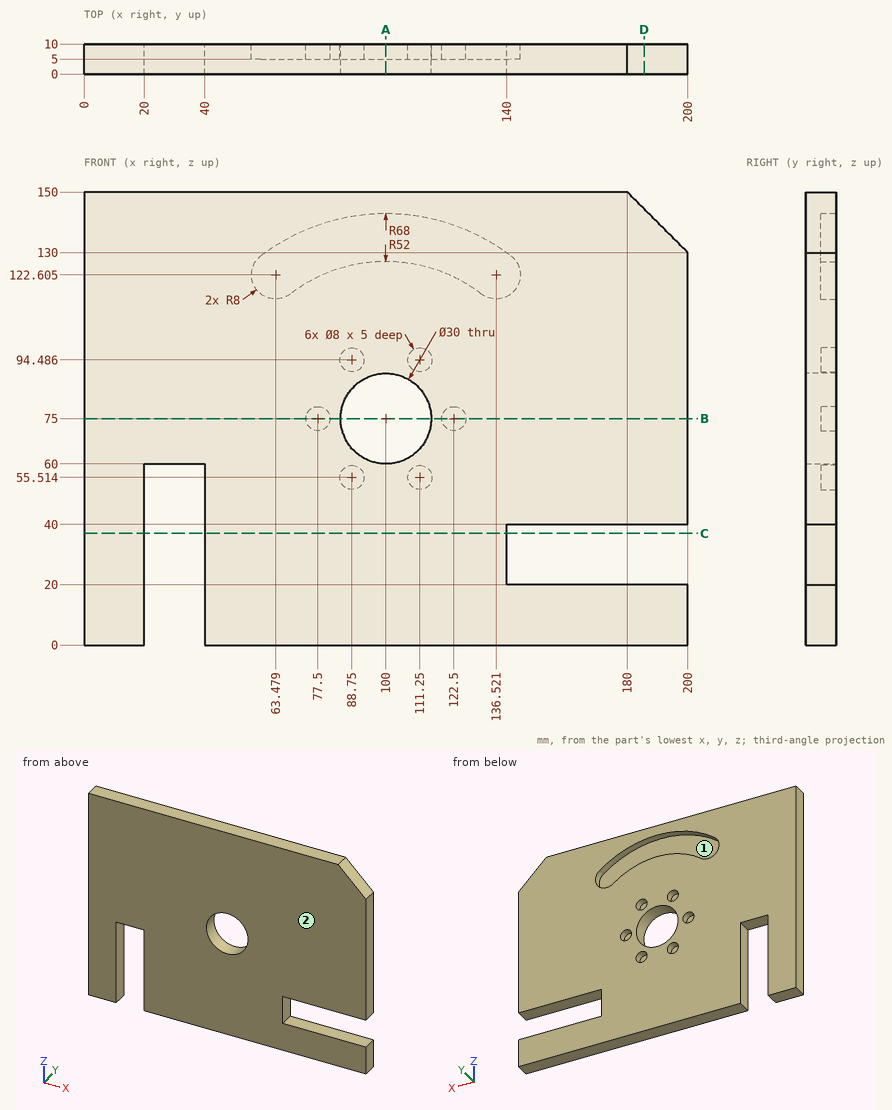
Here's the drawing with two shaded views (mm, measured from the low corner). I have some questions. Round coordinates to 2 decimals unless told otherwise and drop trailing zeros. Loops run counter-clockwise (first coordinate to the right, second up) from the corner with the lowest first, then second, coordinate; pieces in that order, holes last. Notation, with made-up numbers: (51, -18) - (58, -18) arc R24 cw to (58, 14) - close; hole circle Ø3 at (31.25, -13). An arc over 180 degrees is marked (long way). Write item = value, one per line.
1) I need wall thicknesses on line 1 along X through (y, z) = (7.7, 75); line 2 along Z through (x, y) = (164, 5.5); line 3 along Z through (x, y) = (101, 6.75). Which ranges of each line are inside material? Lowest first, please. Write a range as from..to.
Computed:
line_1 = 0..73.5, 81.5..85, 115..118.5, 126.5..200
line_2 = 0..20, 40..150
line_3 = 0..60.03, 89.97..126.99, 142.99..150
2) Imagine slicing it at D-D (x = 185.5). Please give me the cut outline in (y, z).
Computed:
outline = (0, 0) - (10, 0) - (10, 20) - (0, 20) - close; (0, 40) - (10, 40) - (10, 144.5) - (0, 144.5) - close
3) Imagine slicing it at C-C (z = 37). Please give me the cut outline in (x, y), and give its area (3 significant figures).
Computed:
outline = (0, 0) - (20, 0) - (20, 10) - (0, 10) - close; (40, 0) - (140, 0) - (140, 10) - (40, 10) - close
area = 1,200 mm2
4) Imagine slicing it at B-B (z = 75). Please give me the cut outline in (x, y), and give its area (3 significant figures).
Computed:
outline = (0, 0) - (85, 0) - (85, 10) - (81.5, 10) - (81.5, 5) - (73.5, 5) - (73.5, 10) - (0, 10) - close; (115, 0) - (200, 0) - (200, 10) - (126.5, 10) - (126.5, 5) - (118.5, 5) - (118.5, 10) - (115, 10) - close
area = 1,620 mm2
5) I'm going to push flat-ended pins straight in: P1, Ø3, axis at y = 4, z = 34, coming from the +X side; P2, Ø2.5, axis at x = 124, z = 73.5, coming from the +Y side. Where does each tip first touch, or does it pass through?
Computed:
P1 = 140
P2 = 5
6) Imagine slicing it at A-A (x = 100). Please give me the cut outline in (y, z).
Computed:
outline = (0, 0) - (10, 0) - (10, 60) - (0, 60) - close; (0, 90) - (10, 90) - (10, 127) - (5, 127) - (5, 143) - (10, 143) - (10, 150) - (0, 150) - close
7) If we mould it in two halves opening along X, with no side actions, what happens to the marked faces 1 and 2? For each: pulls with the +X half, pulls with the -X half, needs draft (parallel to the pull), parting line crosses it, or undercut.
Computed:
face_1 = undercut
face_2 = needs draft
